```python
from build123d import *

# Parameters (mm, degrees)
F0_W     = 1270
F0_H     = 1270
F1_DEPTH = 1270
F2_R     = 254
F3_DEPTH = 1270.001
F4_SIZE  = 25.4
F5_R     = 25.4
F6_R     = 25.4


with BuildPart() as f1:
    # F0 (on Top) → F1 (new body)
    with BuildSketch(Plane.XY):
        Rectangle(F0_W, F0_H)
    extrude(amount=F1_DEPTH)

    # F2 (on face) → F3 (cut, through all)
    with BuildSketch(Plane.XY.offset(1270)):
        Circle(F2_R)
    extrude(amount=-F3_DEPTH, mode=Mode.SUBTRACT)

    # F4
    f4_edges = [f1.edges().sort_by_distance(p)[0] for p in [
        (0, -635, 1270),
        (-635, 0, 1270),
        (635, 0, 1270),
        (0, 635, 1270),
        (-254, 0, 1270),
    ]]
    chamfer(f4_edges, length=F4_SIZE)

    # F5
    f5_edges = [f1.edges().sort_by_distance(p)[0] for p in [
        (-254, 0, 0),
    ]]
    fillet(f5_edges, radius=F5_R)

    # F6
    f6_edges = [f1.edges().sort_by_distance(p)[0] for p in [
        (0, 635, 0),
    ]]
    fillet(f6_edges, radius=F6_R)

    # F7 (on Front) → F8 (revolve)
    with BuildSketch(Plane.XZ):
        Polygon((-635, 0), (-635, 622.3), (-1143, 622.3), (-1050.3706932068, 354.807138443), (-922.2957491875, 179.8755228519), align=None)
    revolve(axis=Axis((-889, 0, 622.3), (-1, 0, 0)))


solid = f1.part
```
The model under review builds one solid part; all positions refer to its coordinate system, in mm. A direction names the side the tool comes from. Give positions to 0.01 mm unless a question says otherwise; leave off trailing zeros. Write each loop counter-clockwise with the first axis right and the second up, starting at its lowest first coordinate (ties: lowest second). Pieces come first, ordered by that corner, then holes. Notation, with made-up numbers: (80, 50.5) -> (96, 50.5) arc R13 ccw to (96, 65.5) -> close; hole circle Ø2 at (1.5, 67.25). An arc over 180 degrees is marked (long way). Put each result on its own line as item: value.
(1) To check wall thickness, follow probe 1 along Y at (x, z) = (0, 440); probe 2 along X at (y, z) = (132.5, 288.5); probe 3 along X at (y, z) = (115, 382). State the ranges of each line that lie inside material, in increasing order. Write a range as from..to.
Results are:
probe 1: -635..-254, 254..635
probe 2: -983.27..-216.7, 216.7..635
probe 3: -1050.75..-226.48, 226.48..635
(2) We need section B-B, the plane x = -702. Give the boundary of the cut face in (y, z), and give its area (3 significant figures).
Results are:
outline: circle Ø1160.7 at (0, 622.3)
area: 1,060,000 mm²
(3) For pin 1 Ø1.5 at (x, y) = (1.5, -460.5) entering from -Z; pin 2 Ø5 at (x, z) = (-704, 1060) entering from -Y; pin 3 Ø10 at (y, z) = (-490, 759.5) entering from -X; pin 4 Ø10 at (y, z) = (-113, 299) entering from -X, all flat-tipped, find the tip position at first contact; note any pin that passes through.
Results are:
pin 1: z = 0
pin 2: y = -382.9
pin 3: x = -824.19
pin 4: x = -999.13
(4) We need section A-A, the plane x = 0. Give the boundary of the cut face in (y, z).
Results are:
outline: (-635, 0) -> (-279.4, 0) arc R25.4 ccw to (-254, 25.4) -> (-254, 1244.6) -> (-279.4, 1270) -> (-609.6, 1270) -> (-635, 1244.6) -> close; (254, 25.4) arc R25.4 ccw to (279.4, 0) -> (609.6, 0) arc R25.4 ccw to (635, 25.4) -> (635, 1244.6) -> (609.6, 1270) -> (279.4, 1270) -> (254, 1244.6) -> close
(5) The part is to be moulded in two halves that separate along Y. For faces 1 (the flat face through (-9, 635, 626)), 2 (the cylindrical face through (-55.06, -247.96, 643.53)), 3 (the conical face through (-904.32, -19.95, 1075.54)), say which applies: pulls with the +Y half, pulls with the -Y half, needs draft (parallel to the pull), parting line crosses it, or undercut.
Results are:
face 1: pulls with the +Y half
face 2: undercut
face 3: parting line crosses it
(6) Tool access review of faces 4 (the flat face through (-635, 622, 665)), 5 (the flat face through (-635, -625, 619)), 6 (the conical face through (-55.33, -249.16, 1245.83)): name each direction out of +Z, -Z, +X, -X, +Y, -Y from which nothing blocks a thin tool from reaching the whole face with its end or side.
Results are:
face 4: -X, +Y
face 5: -X, -Y
face 6: +Z
